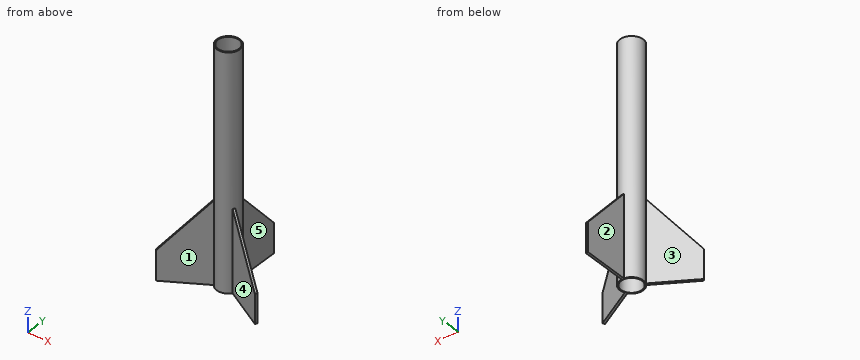
from build123d import *

# Parameters (mm, degrees)
F0_R     = 9
F1_DEPTH = 70
F2_R     = 9
F3_DEPTH = 130
F5_DEPTH = 2
F7_DEPTH = 25
F9_DEPTH = 25


with BuildPart() as f1:
    # F0 (on Top) → F1 (new body)
    with BuildSketch(Plane.XY):
        with BuildLine():
            Line((-1, 49.9498743711), (-1, 9.9498743711))
            ThreePointArc((-1, 9.9498743711), (-8.6602540378, 5), (-9.1168439698, -4.1089117817))
            Line((-9.1168439698, -4.1089117817), (-43.7578601212, -24.1089117817))
            Line((-43.7578601212, -24.1089117817), (-43.2578601212, -24.9749371855))
            Line((-43.2578601212, -24.9749371855), (-42.7578601212, -25.8409625893))
            Line((-42.7578601212, -25.8409625893), (-8.1168439698, -5.8409625893))
            ThreePointArc((-8.1168439698, -5.8409625893), (0, -10), (8.1168439698, -5.8409625893))
            Line((8.1168439698, -5.8409625893), (42.7578601212, -25.8409625893))
            Line((42.7578601212, -25.8409625893), (43.2578601212, -24.9749371855))
            Line((43.2578601212, -24.9749371855), (43.7578601212, -24.1089117817))
            Line((43.7578601212, -24.1089117817), (9.1168439698, -4.1089117817))
            ThreePointArc((9.1168439698, -4.1089117817), (8.6602540378, 5), (1, 9.9498743711))
            Line((1, 9.9498743711), (1, 49.9498743711))
            Line((1, 49.9498743711), (0, 49.9498743711))
            Line((0, 49.9498743711), (-1, 49.9498743711))
        make_face()
        Circle(F0_R, mode=Mode.SUBTRACT)
    extrude(amount=F1_DEPTH)

    # F2 (on face) → F3 (join)
    with BuildSketch(Plane.XY.offset(70)):
        with BuildLine():
            ThreePointArc((9.1168439698, -4.1089117817), (9.7767182556, -2.1013757758), (10, 0))
            ThreePointArc((10, 0), (7.4161984871, 6.7082039325), (1, 9.9498743711))
            ThreePointArc((1, 9.9498743711), (0, 10), (-1, 9.9498743711))
            ThreePointArc((-1, 9.9498743711), (-8.6602540378, 5), (-9.1168439698, -4.1089117817))
            ThreePointArc((-9.1168439698, -4.1089117817), (-8.6602540378, -5), (-8.1168439698, -5.8409625893))
            ThreePointArc((-8.1168439698, -5.8409625893), (0, -10), (8.1168439698, -5.8409625893))
            ThreePointArc((8.1168439698, -5.8409625893), (8.6602540378, -5), (9.1168439698, -4.1089117817))
        make_face()
        Circle(F2_R, mode=Mode.SUBTRACT)
    extrude(amount=F3_DEPTH)

    # F4 (on face) → F5 (cut, through all)
    with BuildSketch(Plane.YZ.offset(1)):
        Polygon((49.9498743711, 70), (9.9498743711, 70), (49.9498743711, 25), align=None)
    extrude(amount=-F5_DEPTH, mode=Mode.SUBTRACT)

    # F6 (on face) → F7 (cut)
    with BuildSketch(Plane(origin=(0.5, 0.8660254038, 0), x_dir=(-0.8660254038, 0.5, 0), z_dir=(0.5, 0.8660254038, 0))):
        Polygon((-49.9498743711, 25), (-9.9498743711, 70), (-49.9498743711, 70), align=None)
    extrude(amount=-F7_DEPTH, mode=Mode.SUBTRACT)

    # F8 (on face) → F9 (cut)
    with BuildSketch(Plane(origin=(-0.5, 0.8660254038, 0), x_dir=(-0.8660254038, -0.5, 0), z_dir=(-0.5, 0.8660254038, 0))):
        Polygon((49.9498743711, 70), (9.9498743711, 70), (49.9498743711, 25), align=None)
    extrude(amount=-F9_DEPTH, mode=Mode.SUBTRACT)


solid = f1.part
Input: part model. Units: mm. Frame: model coordinates. Face numbers are marked on the shaded views. A direction names the side the tool comes from. Coordinates: 2 decimals unless noted, no trailing zeros. Loops run counter-clockwise (first coordinate to the right, second up) from the corner with the lowest first, then second, coordinate; pieces in that order, holes last. Notation, with made-up numbers: (79.5, -1) -> (133.5, -1) arc R6 ccw to (133.5, 10) -> close; hole circle Ø7 at (-32, 60). An arc over 180 degrees is marked (long way). Write each question's results on one line, items separated by ' | '. Start each with the question number.
Q1. Section D-D, the plane z = 50.5. Return the cut outline in (x, y).
Q2. Ray query, line 1 (X direction, y = 8, z = 150); line 2 (X direction, y = 33, z = 27); line 3 (Y direction, x = 6, z = 45). Return the intervals inside material, ascending. Write a range as from..to.
Q3. Section A-A, the plane z = 18. Return the cut outline in (x, y).
Q4. Section C-C, the plane x = 6. Return the cut outline in (y, z).
Q5. Section B-B, the plane y = 0. Return the cut outline in (x, z), plus the area to 3 significant figures.
Q6. Pin query (flat end, axial travel): pin 1 (20 mm diameter, centred on y = 23.5, z = 40.5, fed in from +X); pin 2 (3 mm diameter, centred on x = 3.5, z = 154.5, fed in from +Y); pin 3 (0.8 mm diameter, centred on x = 8.5, y = -5, fed in from -Z); pin 4 (3 mm diameter, centred on y = 6.5, z = 171, fed in from +X). Return the tip coordinate at first contact, or that it passes through.
Q7. Reachability of the marked faces 1 and 2 from +Z, -Z, +X, -X, +Y, -Y: full face, straight path, thin tool, end or side. Return the list, or none.
Q8. Pull-direction query (X, two-part tool) for the marked faces 3, 4 and 5; classes: released by +X, released by -X, zero draft, split by the parting line, or undercut.
Found:
1) outline: (-24.13, -12.78) -> (-23.13, -14.51) -> (-8.12, -5.84) arc R10 ccw to (8.12, -5.84) -> (23.13, -14.51) -> (24.13, -12.78) -> (9.12, -4.11) arc R10 ccw to (1, 9.95) -> (1, 27.28) -> (-1, 27.28) -> (-1, 9.95) arc R10 ccw to (-9.12, -4.11) -> close; hole circle Ø18 at (0, 0)
2) line 1: -6..-4.12, 4.12..6 | line 2: -1..1 | line 3: -8..-6.71, 6.71..8
3) outline: (-43.76, -24.11) -> (-42.76, -25.84) -> (-8.12, -5.84) arc R10 ccw to (8.12, -5.84) -> (42.76, -25.84) -> (43.76, -24.11) -> (9.12, -4.11) arc R10 ccw to (1, 9.95) -> (1, 49.95) -> (-1, 49.95) -> (-1, 9.95) arc R10 ccw to (-9.12, -4.11) -> close; hole circle Ø18 at (0, 0)
4) outline: (-8, 0) -> (-6.71, 0) -> (-6.71, 200) -> (-8, 200) -> close; (6.71, 0) -> (8, 0) -> (8, 200) -> (6.71, 200) -> close
5) outline: (-10, 0) -> (-9, 0) -> (-9, 200) -> (-10, 200) -> close; (9, 0) -> (10, 0) -> (10, 200) -> (9, 200) -> close | area: 400 mm2
6) pin 1: x = 1 | pin 2: y = 9.8 | pin 3: z = 0 | pin 4: x = 8.66
7) face 1: +Z, -Z, -Y | face 2: +Z, -Z, -X, +Y
8) face 3: released by -X | face 4: undercut | face 5: released by +X
